from build123d import *

# Parameters (mm, degrees)
BOSS_EXTRUDE4_DEPTH = 200
SHELL2_T            = -3
SKETCH4_R           = 8.02
BOSS_EXTRUDE5_DEPTH = 3
SKETCH4_7_R         = 8.02
CUT_EXTRUDE1_DEPTH  = 4
CUT_EXTRUDE2_START  = 4
SKETCH5_R           = 8.02
CUT_EXTRUDE2_DEPTH  = 4


with BuildPart() as part:
    # Sketch1 → Boss-Extrude4 (new body)
    with BuildSketch(Plane.XY):
        Polygon((0, 0), (200, 0), (200, 80), (180, 80), align=None)
    extrude(amount=BOSS_EXTRUDE4_DEPTH)

    # Shell2
    shell2_openings = [part.faces().sort_by_distance(p)[0] for p in [
        (90, 40, 100),
    ]]
    offset(amount=SHELL2_T, openings=shell2_openings, kind=Kind.INTERSECTION)

    # Sketch4 → Boss-Extrude5 (add)
    with BuildSketch(Plane.XY.offset(200)):
        with Locations((91.379034553, 20)):
            Circle(SKETCH4_R)
        with Locations((118.899034553, 20)):
            Circle(SKETCH4_R)
    extrude(amount=-BOSS_EXTRUDE5_DEPTH)

    # Sketch4<7> → Cut-Extrude1 (cut)
    with BuildSketch(Plane.XY.offset(200)):
        with Locations((91.379034553, 20)):
            Circle(SKETCH4_7_R)
        with Locations((118.899034553, 20)):
            Circle(SKETCH4_7_R)
    extrude(amount=-CUT_EXTRUDE1_DEPTH, mode=Mode.SUBTRACT)

    # Sketch5 → Cut-Extrude2 (cut)
    with BuildSketch(Plane.XY.offset(CUT_EXTRUDE2_START)):
        with Locations((91.379034553, 20)):
            Circle(SKETCH5_R)
        with Locations((118.899034553, 20)):
            Circle(SKETCH5_R)
    extrude(amount=-CUT_EXTRUDE2_DEPTH, mode=Mode.SUBTRACT)


solid = part.part
Build history of the part. All positions in model axes, mm. A direction names the side the tool comes from. Round coordinates to 2 decimals unless told otherwise and drop trailing zeros. Write each loop counter-clockwise with the first axis right and the second up, starting at its lowest first coordinate (ties: lowest second). Pieces come first, ordered by that corner, then holes. Notation, with made-up numbers: M 61.5,48.5 L 92.5,48.5 A21 ccw 92.5,68.5 Z; hole C 34,68.25 d2. An arc over 180 degrees is marked long. Answer in a Markdown table with one row per item.
1. Mould opens along Y. For faces 3 (the face through (3.753, 1.668, 99.533)), 4 (the face through (197, 39, 99)), 5 (the face through (143, 32, 0)) say: +Y half, -Y half, draft (parallel to the pull), parting line (faces both ways), or undercut.
Geometry check:
| item | result |
|---|---|
| face 3 | +Y half |
| face 4 | undercut |
| face 5 | draft |
2. Saw through at C-C (y = 7). List the corners of the cut face in (x, z), and give its area (3 significant figures).
Geometry check:
| item | result |
|---|---|
| outline | M 15.75,0 L 200,0 L 200,200 L 15.75,200 L 15.75,197 L 197,197 L 197,3 L 15.75,3 Z |
| area | 1,690 mm2 |
3. Saw through at B-B (z = 146.5). List the corners of the cut face in (x, y), and give its area (3 significant figures).
Geometry check:
| item | result |
|---|---|
| outline | M 0,0 L 200,0 L 200,80 L 180,80 L 173.25,77 L 197,77 L 197,3 L 6.75,3 Z |
| area | 882 mm2 |
4. Flat gauge pins, fed straight in: P1, Ø12, axis at x = 54.5, z = 78.5, coming from the +Y side; P2, Ø7, axis at x = 180, z = 130.5, coming from the -Y side; P3, Ø22, axis at y = 56.5, z = 95.5, coming from the -X side. Where does each tip first touch, or does it go through?
Geometry check:
| item | result |
|---|---|
| P1 | y = 3 |
| P2 | y = 0 |
| P3 | x = 197 |
5. Which spindle directions (+Z, -Z, +X, -X, +Y, -Y) get a long thin tool onto all of the face, cutting with end or side? Do faces 1 (the face through (200, 39, 99)), 2 (the face through (122, 32, 3)). Say none if no direction does.
Geometry check:
| item | result |
|---|---|
| face 1 | +Z, -Z, +X, +Y, -Y |
| face 2 | -X |
6. Saw through at A-A (y = 20). List the corners of the cut face in (x, z), and give its area (3 significant figures).
Geometry check:
| item | result |
|---|---|
| outline | M 45,0 L 83.36,0 L 83.36,3 L 45,3 Z; M 45,197 L 83.36,197 L 83.36,200 L 45,200 Z; M 99.4,0 L 110.88,0 L 110.88,3 L 99.4,3 Z; M 99.4,197 L 110.88,197 L 110.88,200 L 99.4,200 Z; M 126.92,0 L 200,0 L 200,200 L 126.92,200 L 126.92,197 L 197,197 L 197,3 L 126.92,3 Z |
| area | 1,320 mm2 |
7. Probe L1, parallel to Z at x = 183.5, y = 73.5; L2, parallel to Y at x = 182, z = 178; L3, parallel to X at y = 37.5, z = 173. List the from-to ranges inside material, lowest first. Write a range as [from, to].
Geometry check:
| item | result |
|---|---|
| L1 | [0, 3], [197, 200] |
| L2 | [0, 3], [77, 80] |
| L3 | [197, 200] |
